```python
from build123d import *

# Parameters (mm, degrees)
SKETCH_1_W          = 20
SKETCH_1_H          = 41
SKETCH_1_R          = 1.3
EXTRUDE_1_DEPTH     = 2
SKETCH_1_3_W        = 1.5
SKETCH_1_3_H        = 41
EXTRUDE_2_DEPTH     = 25
SKETCH_2_R          = 1.2
SKETCH_2_R_2        = 6.4
CUT_EXTRUDE_1_DEPTH = 22.5
EXTRUDE_6_DEPTH     = 25
SKETCH_4_W          = 20
SKETCH_4_H          = 2
EXTRUDE_8_DEPTH     = 1.5


with BuildPart() as part:
    # Sketch 1 → Extrude 1 (new body)
    with BuildSketch(Plane.XY):
        Rectangle(SKETCH_1_W, SKETCH_1_H)
        with Locations((-4.949747468, 4.949747468)):
            Circle(SKETCH_1_R, mode=Mode.SUBTRACT)
        with Locations((-7, 0)):
            Circle(SKETCH_1_R, mode=Mode.SUBTRACT)
        with Locations((-4.949747468, -4.949747468)):
            Circle(SKETCH_1_R, mode=Mode.SUBTRACT)
        with Locations((0, -7)):
            Circle(SKETCH_1_R, mode=Mode.SUBTRACT)
        with Locations((4.949747468, -4.949747468)):
            Circle(SKETCH_1_R, mode=Mode.SUBTRACT)
        with Locations((7, 0)):
            Circle(SKETCH_1_R, mode=Mode.SUBTRACT)
        with Locations((4.949747468, 4.949747468)):
            Circle(SKETCH_1_R, mode=Mode.SUBTRACT)
        with Locations((0, 7)):
            Circle(SKETCH_1_R, mode=Mode.SUBTRACT)
    extrude(amount=EXTRUDE_1_DEPTH)

    # Sketch 1_3 → Extrude 2 (add)
    with BuildSketch(Plane.XY):
        with Locations((10.75, 0)):
            Rectangle(SKETCH_1_3_W, SKETCH_1_3_H)
    extrude(amount=EXTRUDE_2_DEPTH)

    # Sketch 2 → Cut-Extrude 1 (cut, through all)
    with BuildSketch(Plane(origin=(11.5, 0, 0), x_dir=(0, 0, -1), z_dir=(1, 0, 0))):
        with Locations((-22.5, -18)):
            Circle(SKETCH_2_R)
        with Locations((-6.5, -18)):
            Circle(SKETCH_2_R)
        with Locations((-22.5, 18)):
            Circle(SKETCH_2_R)
        with Locations((-6.5, 18)):
            Circle(SKETCH_2_R)
        with Locations((-14.5, -10)):
            Circle(SKETCH_2_R_2)
    extrude(amount=-CUT_EXTRUDE_1_DEPTH, mode=Mode.SUBTRACT)

    # Sketch 1_6 → Extrude 6 (add)
    with BuildSketch(Plane.XY):
        Polygon((-10, 20.5), (-10, 22.5), (11.5, 22.5), (11.5, 20.5), (10, 20.5), align=None)
    extrude(amount=EXTRUDE_6_DEPTH)

    # Sketch 4 → Extrude 8 (add)
    with BuildSketch(Plane.XY.offset(2)):
        with Locations((0, -19.5)):
            Rectangle(SKETCH_4_W, SKETCH_4_H)
    extrude_8 = extrude(amount=EXTRUDE_8_DEPTH)

    # Mirror 1: Extrude 8 across plane
    add(extrude_8.mirror(Plane.ZX))


solid = part.part
```
Read the model definition and answer for the solid it produces. Units are mm, in the model's axes. A direction names the side the tool comes from. Give positions to 0.01 mm unless a question says otherwise; leave off trailing zeros. Loops run counter-clockwise (first coordinate to the right, second up) from the corner with the lowest first, then second, coordinate; pieces in that order, holes last.
Item 1: The part is cut by section A-A (y = 7). Write down the section's boundary in (x, z).
Item 2: For faces 1 (the flat face through (0, 19, 3.5)), 2 (the cylindrical face through (-0.28, -8.27, 0.99)), 3 (the flat face through (0, -18.5, 3)), determine the directions among +Z, -Z, +X, -X, +Y, -Y from which every point of the face is accessible in a straight line to the end or side of a thin tool.
Item 3: The part is cut by section C-C (y = 0.5). Write down the section's boundary in (x, z).
Item 4: The part is cut by section D-D (x = 0). Write down the section's boundary in (y, z), and give its area (3 significant figures).
Item 5: Each of these flat-tipped pins is pushed along its axis until it touches: pin 1 Ø3 at (y, z) = (18, 6.5) entering from -X; pin 2 Ø1.6 at (x, y) = (-4.95, -4.95) entering from -Z; pin 3 Ø10 at (x, y) = (1.5, -9) entering from +Z; pin 4 Ø4 at (x, z) = (1, 7.5) entering from -Y. Where does it stop, or does it pass through?
Item 6: The part is cut by section B-B (z = 6.5). Write down the section's boundary in (x, y), and give its area (3 significant figures).
Item 7: Find the intervals of material crossed by line 1 along Z through (x, y) = (-5, -9); line 2 along X through (y, z) = (-5, 22.75); line 3 along Y through (x, z) = (8, 8.25), in increasing order.
Item 8: The mould has two halves that part along X. Classify faces 4 (the flat face through (-10, 7, 1)), 5 (the cylindrical face through (-4.35, -6.103, 0.986)), 6 (the flat face through (11.5, 1, 12)), 7 (the cylindrical face through (4.67, -6.22, 0.99)): released by +X, released by -X, zero draft, split by the parting line, or undercut.
Taken from the geometry:
1. outline: (-10, 0) - (-1.3, 0) - (-1.3, 2) - (-10, 2) - close; (1.3, 0) - (11.5, 0) - (11.5, 25) - (10, 25) - (10, 2) - (1.3, 2) - close
2. face 1: +Z, -X, -Y
2. face 2: +Z, -Z
2. face 3: +Z, -X
3. outline: (-10, 0) - (-8.2, 0) - (-8.2, 2) - (-10, 2) - close; (-5.8, 0) - (5.8, 0) - (5.8, 2) - (-5.8, 2) - close; (8.2, 0) - (11.5, 0) - (11.5, 25) - (10, 25) - (10, 2) - (8.2, 2) - close
4. outline: (-20.5, 0) - (-8.3, 0) - (-8.3, 2) - (-18.5, 2) - (-18.5, 3.5) - (-20.5, 3.5) - close; (-5.7, 0) - (5.7, 0) - (5.7, 2) - (-5.7, 2) - close; (8.3, 0) - (22.5, 0) - (22.5, 25) - (20.5, 25) - (20.5, 3.5) - (18.5, 3.5) - (18.5, 2) - (8.3, 2) - close
4. area: 128 mm2
5. pin 1: stops at x = 10
5. pin 2: passes through
5. pin 3: stops at z = 2
5. pin 4: stops at y = 20.5
6. outline: (-10, 20.5) - (10, 20.5) - (10, 19.2) - (11.5, 19.2) - (11.5, 22.5) - (-10, 22.5) - close; (10, -20.5) - (11.5, -20.5) - (11.5, -19.2) - (10, -19.2) - close; (10, -16.8) - (11.5, -16.8) - (11.5, 16.8) - (10, 16.8) - close
6. area: 97.3 mm2
7. line 1: z = 0 to 2
7. line 2: x = 10 to 11.5
7. line 3: y = 20.5 to 22.5
8. face 4: released by -X
8. face 5: undercut
8. face 6: released by +X
8. face 7: undercut
